Source: three-view drawing plus pictorial views. Frame: mm from the lowest corner of the part. Round coordinates to 2 decimals unless told otherwise and drop trailing zeros. Answer in a Markdown table with one row per item.
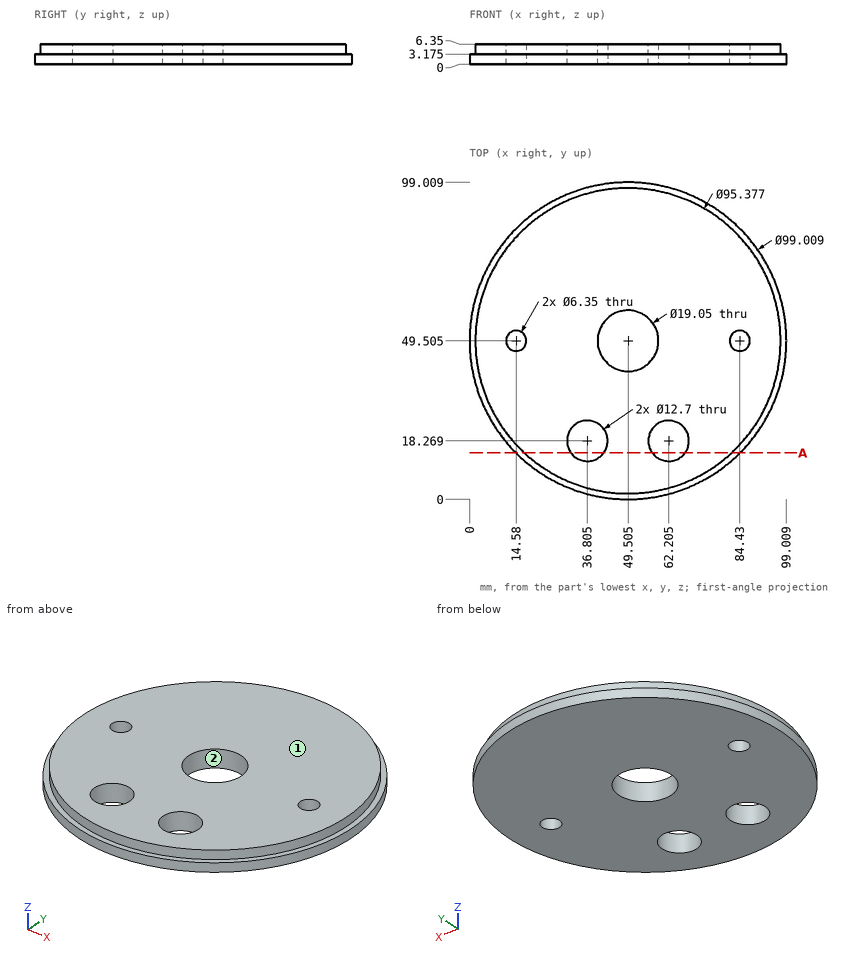
Q1. Pull-direction query (Y, two-part tool) for the marked faces 1 and 2; classes: pulls with the +Y half, pulls with the -Y half, needs draft (parallel to the pull), parting line crosses it, or undercut.
Solutions:
| item | result |
|---|---|
| face 1 | needs draft |
| face 2 | undercut |
Q2. Contact query for flat-ended pins moving along their axis: pin 1 Ø1 at (y, z) = (31.5, 5.5) entering from -X (1 decimal); pin 2 Ø1.5 at (y, z) = (26.5, 4) entering from +X; pin 3 Ø2 at (y, z) = (78.5, 3.5) entering from +X (1 decimal). Output: stop coordinate, or through.
Solutions:
| item | result |
|---|---|
| pin 1 | stops at x = 5.1 |
| pin 2 | stops at x = 91.68 |
| pin 3 | stops at x = 90.3 |
Q3. Section A-A (y = 14.5). State how many separate pieces and enclosed holes the cut face has, and give its area (3 significant figures).
Solutions:
| item | result |
|---|---|
| separate pieces | 3 |
| enclosed holes | 0 |
| area | 298 mm2 |
Q4. Material intervals for probe 1 along X at (y, z) = (19.5, 5.25) (1 decimal); probe 2 along Y at (x, z) = (65, 2); probe 3 along Y at (x, z) = (52, 5.5), sorted ascending.
Solutions:
| item | result |
|---|---|
| probe 1 | x = 12.4 to 30.6, 43 to 56, 68.4 to 86.6 |
| probe 2 | y = 2.49 to 12.57, 23.97 to 96.52 |
| probe 3 | y = 1.88 to 40.31, 58.7 to 97.13 |
